Geometry check sheet. Reference: the model listing, model coordinates, mm. Face numbers are marked on the shaded views. A direction names the side the tool comes from. Coordinates: 2 decimals unless noted, no trailing zeros. Loops run counter-clockwise (first coordinate to the right, second up) from the corner with the lowest first, then second, coordinate; pieces in that order, holes last. Notation, with made-up numbers: (61.5, -10.75) -> (113.5, -10.75) arc R30 cw to (113.5, 14.25) -> close; hole circle Ø6 at (17, 47.25). An arc over 180 degrees is marked (long way). Answer as a JSON object with one key per item and string values.
from build123d import *

# Parameters (mm, degrees)
SKETCH1_W           = 60
SKETCH1_H           = 40
BOSS_EXTRUDE1_DEPTH = 240
SKETCH2_W           = 25
SKETCH2_H           = 40
CUT_EXTRUDE1_DEPTH  = 35
BOSS_EXTRUDE7_DEPTH = 25
BOSS_EXTRUDE5_START = 25
BOSS_EXTRUDE5_DEPTH = 25
SKETCH3_W           = 30
SKETCH3_H           = 20
BOSS_EXTRUDE2_DEPTH = 35
SKETCH5_R           = 2.5
CUT_EXTRUDE3_DEPTH  = 30
CUT_EXTRUDE4_DEPTH  = 240
CUT_EXTRUDE5_DEPTH  = 20
CUT_EXTRUDE6_DEPTH  = 25
CUT_EXTRUDE7_START  = -25
CUT_EXTRUDE7_DEPTH  = 25
SKETCH19_R          = 2.5
CUT_EXTRUDE8_DEPTH  = 30
CUT_EXTRUDE9_DEPTH  = 30


with BuildPart() as part:
    # Sketch1 → Boss-Extrude1 (new body)
    with BuildSketch(Plane.XY):
        with Locations((-30, 20)):
            Rectangle(SKETCH1_W, SKETCH1_H)
    extrude(amount=BOSS_EXTRUDE1_DEPTH)

    # Sketch2 → Cut-Extrude1 (cut)
    with BuildSketch(Plane(origin=(0, 40, 0), x_dir=(1, 0, 0), z_dir=(0, 1, 0))):
        with Locations((-47.5, -220)):
            Rectangle(SKETCH2_W, SKETCH2_H)
        with Locations((-12.5, -220)):
            Rectangle(SKETCH2_W, SKETCH2_H)
    extrude(amount=-CUT_EXTRUDE1_DEPTH, mode=Mode.SUBTRACT)

    # Sketch18 → Boss-Extrude7 (add)
    with BuildSketch(Plane(origin=(-25, 0, 0), x_dir=(0, 0, -1), z_dir=(1, 0, 0))):
        with BuildLine():
            Line((-200, 5), (-210, 5))
            ThreePointArc((-210, 5), (-202.928932188, 7.928932188), (-200, 15))
            Line((-200, 15), (-200, 5))
        make_face()
    extrude(amount=BOSS_EXTRUDE7_DEPTH)

    # Sketch16 → Boss-Extrude5 (add)
    with BuildSketch(Plane.ZY.offset(35).offset(BOSS_EXTRUDE5_START)):
        with BuildLine():
            Line((200, 15), (160, 5))
            Line((160, 5), (210, 5))
            ThreePointArc((210, 5), (202.928932188, 7.928932188), (200, 15))
        make_face()
    extrude(amount=-BOSS_EXTRUDE5_DEPTH)

    # Sketch3 → Boss-Extrude2 (add)
    with BuildSketch(Plane(origin=(0, 40, 0), x_dir=(1, 0, 0), z_dir=(0, 1, 0))):
        with Locations((-30, -10)):
            Rectangle(SKETCH3_W, SKETCH3_H)
    extrude(amount=BOSS_EXTRUDE2_DEPTH)

    # Sketch5 → Cut-Extrude3 (cut)
    with BuildSketch(Plane(origin=(-25, 0, 0), x_dir=(0, 0, -1), z_dir=(1, 0, 0))):
        with Locations(Location((-220, 25, 0), (0, 0, 90))):
            Circle(SKETCH5_R)
    extrude(amount=-CUT_EXTRUDE3_DEPTH, mode=Mode.SUBTRACT)

    # Sketch6 → Cut-Extrude4 (cut)
    with BuildSketch(Plane(origin=(0, 0, 0), x_dir=(-1, 0, 0), z_dir=(0, 0, -1))):
        with BuildLine():
            Line((60, 20), (60, 0))
            Line((60, 0), (40, 0))
            ThreePointArc((40, 0), (54.142135624, 5.857864376), (60, 20))
        make_face()
        with BuildLine():
            Line((0, 20), (0, 0))
            Line((0, 0), (20, 0))
            ThreePointArc((20, 0), (5.857864376, 5.857864376), (0, 20))
        make_face()
    extrude(amount=-CUT_EXTRUDE4_DEPTH, mode=Mode.SUBTRACT)

    # Sketch8 → Cut-Extrude5 (cut)
    with BuildSketch(Plane(origin=(-25, 0, 0), x_dir=(0, 0, -1), z_dir=(1, 0, 0))):
        with BuildLine():
            Line((-240, 40), (-240, 22.5))
            ThreePointArc((-240, 22.5), (-234.537682266, 34.537682266), (-222.5, 40))
            Line((-222.5, 40), (-240, 40))
        make_face()
    extrude(amount=-CUT_EXTRUDE5_DEPTH, mode=Mode.SUBTRACT)

    # Sketch10 → Cut-Extrude6 (cut)
    with BuildSketch(Plane(origin=(0, 0, 0), x_dir=(0, 0, -1), z_dir=(1, 0, 0))):
        with BuildLine():
            Line((-200, 40), (-195, 40))
            ThreePointArc((-195, 40), (-198.535533906, 38.535533906), (-200, 35))
            Line((-200, 35), (-200, 40))
        make_face()
    extrude(amount=-CUT_EXTRUDE6_DEPTH, mode=Mode.SUBTRACT)

    # Sketch11 → Cut-Extrude7 (cut)
    with BuildSketch(Plane.ZY.offset(60).offset(CUT_EXTRUDE7_START)):
        with BuildLine():
            Line((200, 40), (195, 40))
            ThreePointArc((195, 40), (198.535533906, 38.535533906), (200, 35))
            Line((200, 35), (200, 40))
        make_face()
    extrude(amount=CUT_EXTRUDE7_DEPTH, mode=Mode.SUBTRACT)

    # Sketch19 → Cut-Extrude8 (cut)
    with BuildSketch(Plane(origin=(-15, 0, 0), x_dir=(0, 0, -1), z_dir=(1, 0, 0))):
        with Locations((-10, 60)):
            Circle(SKETCH19_R)
    extrude(amount=-CUT_EXTRUDE8_DEPTH, mode=Mode.SUBTRACT)

    # Sketch20 → Cut-Extrude9 (cut)
    with BuildSketch(Plane(origin=(-15, 0, 0), x_dir=(0, 0, -1), z_dir=(1, 0, 0))):
        with BuildLine():
            Line((-20, 75), (0, 75))
            Line((0, 75), (0, 60))
            ThreePointArc((0, 60), (-10, 70), (-20, 60))
            Line((-20, 60), (-20, 75))
        make_face()
    extrude(amount=-CUT_EXTRUDE9_DEPTH, mode=Mode.SUBTRACT)


solid = part.part
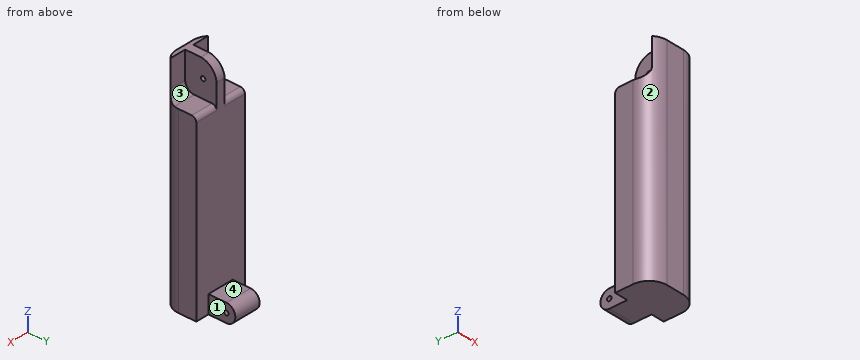
1. Depth check by flat-ended pin: P1, Ø16, axis at x = -53, y = 26, coming from the +Z side; P2, Ø1.5, axis at x = -20.5, y = 39.5, coming from the +Z side; P3, Ø20, axis at x = -19, z = 228, coming from the +Y side. Enter the tip coordinate at first touch or a pass-through.
Evaluation:
{"P1": "stops at z = 200", "P2": "stops at z = 198.31", "P3": "stops at y = 40"}
2. Thickness scan on probe 1 along Y at (x, z) = (-33.5, 10); probe 2 along Y at (x, z) = (-32.25, 220); probe 3 along Z at (x, y) = (-13.5, 18.5). Record the ranges inside material, lowest first. Write a range as from..to.
Evaluation:
{"probe 1": "y = 0..57.5, 62.5..70", "probe 2": "y = 0..22.5, 27.5..40", "probe 3": "z = 0..200"}
3. Section check C-C, the plane z = 28. Record the boundary of the cut face in (x, y).
Evaluation:
{"outline": "(-60, 20) arc R20 ccw to (-40, 0) -> (-20, 0) arc R20 ccw to (0, 20) -> (0, 40) -> (-60, 40) -> close"}
4. Section check B-B, the plane x = -17.5. Record the boundary of the cut face in (y, z).
Evaluation:
{"outline": "(0.16, 0) -> (60, 0) arc R10 ccw to (60, 20) -> (40, 20) -> (40, 195) arc R5 ccw to (35, 200) -> (15, 200) arc R10 cw to (5, 210) -> (5, 240) -> (0.16, 240) -> close; hole circle Ø5 at (60, 10)"}
5. Section check D-D, the plane y = 25. Record the boundary of the cut face in (x, z).
Evaluation:
{"outline": "(-60, 0) -> (0, 0) -> (0, 200) -> (-25, 200) -> (-25, 217.5) -> (-35, 217.5) -> (-35, 200) -> (-60, 200) -> close; (-35, 222.5) -> (-25, 222.5) -> (-25, 239.66) -> (-35, 239.66) -> close"}
6. Tool access check on the marked faces 1, 2, 3 and 4. Record the directions out of +Z, -Z, +X, -X, +Y, -Y that give a thin tool (end or side, any length) a straight path to the whole face; none if there is none.
Evaluation:
{"face 1": "+Z, -Z, +X, +Y", "face 2": "+Z, -Z, -X, -Y", "face 3": "+Z, +X, +Y", "face 4": "+Z, +X, -X, +Y"}
7. Section check A-A, the plane z = 220. Record the boundary of the cut face in (x, y), then the cut area to 3 significant figures.
Evaluation:
{"outline": "(-53.23, 5) arc R20 ccw to (-40, 0) -> (-20, 0) arc R20 ccw to (-6.77, 5) -> (-25, 5) -> (-25, 22.5) -> (-35, 22.5) -> (-35, 5) -> close; (-35, 27.5) -> (-25, 27.5) -> (-25, 40) -> (-35, 40) -> close", "area": "491 mm^2"}
